Autodesk Inventor part; units mm, degrees
ref_plane "YZ Plane" through (0, 0, 0) normal (1, 0, 0) x (0, 1, 0)
ref_plane "XZ Plane" through (0, 0, 0) normal (0, 1, 0) x (-1, 0, 0)
ref_plane "XY Plane" through (0, 0, 0) normal (0, 0, 1) x (1, 0, 0)
sketch "Sketch1" plane through (0, 0, 0) normal (0, 0, 1) x (1, 0, 0)
  circle A0 centre (0, 0) radius 30
  dimension "d0" = 60
extrude "Extrusion1" add sketch "Sketch1" along normal blind 5
sketch "Sketch2" plane through (0, 0, 5) normal (0, 0, 1) x (1, 0, 0)
  circle A0 centre (0, 0) radius 24.95
  dimension "d3" = 49.9
extrude "Extrusion2" add sketch "Sketch2" along normal blind 5
sketch "Sketch3" plane through (0, 0, 10) normal (0, 0, 1) x (1, 0, 0)
  circle A0 centre (0, 0) radius 15
  dimension "d6" = 30
extrude "Extrusion3" cut sketch "Sketch3" against normal through all
sketch "Sketch4" plane through (0, 0, 0) normal (0, 0, -1) x (-1, 0, 0)
  circle A0 centre (0, 0) radius 20
  dimension "d9" = 40
extrude "Extrusion4" add sketch "Sketch4" against normal blind 5
sketch "Sketch5" plane through (0, 0, 0) normal (0, 0, -1) x (-1, 0, 0)
  circle A0 centre (0, 0) radius 3.5
  dimension "d12" = 7
extrude "Extrusion5" cut sketch "Sketch5" against normal through all
sketch "Sketch6" plane through (0, 0, 5) normal (0, 0, 1) x (1, 0, 0)
  circle A0 centre (7, 0) radius 1.05
  point P0 (0, 0)
  dimension "d15" = 2.1
  dimension "d16" = 7
extrude "Extrusion6" cut sketch "Sketch6" against normal through all
pattern_circular "Circular Pattern1" count 8 over 360 about axis through (0, 0, -10) along (0, 0, 1) of "Extrusion6"
sketch "Sketch9" plane through (0, 0, 0) normal (0, 0, -1) x (-1, 0, 0)
  circle A0 centre (0, 0) radius 15
  circle A1 centre (-4.9497, -4.9497) radius 1.05
  circle A2 centre (0, -7) radius 1.05
  circle A3 centre (4.9497, -4.9497) radius 1.05
  circle A4 centre (7, 0) radius 1.05
  circle A5 centre (4.9497, 4.9497) radius 1.05
  circle A6 centre (0, 7) radius 1.05
  circle A7 centre (-4.9497, 4.9497) radius 1.05
  circle A8 centre (-7, 0) radius 1.05
  circle A9 centre (0, 0) radius 3.5
  circle A10 centre (0, 0) radius 30
  dimension "d35" = 30
extrude "Extrusion9" cut sketch "Sketch9" against normal through all contours A10
sketch "Sketch10" plane through (0, 0, 5) normal (0, 0, 1) x (1, 0, 0)
  circle A0 centre (0, 0) radius 10
  circle A1 centre (4.9497, -4.9497) radius 1.05
  circle A2 centre (0, -7) radius 1.05
  circle A3 centre (-4.9497, -4.9497) radius 1.05
  circle A4 centre (-7, 0) radius 1.05
  circle A5 centre (-4.9497, 4.9497) radius 1.05
  circle A6 centre (0, 7) radius 1.05
  circle A7 centre (4.9497, 4.9497) radius 1.05
  circle A8 centre (7, 0) radius 1.05
  circle A9 centre (0, 0) radius 3.5
  circle A10 centre (0, 0) radius 15
  dimension "d38" = 20
extrude "Extrusion10" add sketch "Sketch10" along normal blind 5 contours A10
sketch "Sketch11" plane through (0, 0, 0) normal (0, 0, -1) x (-1, 0, 0)
  line L0 (-7.5, 0) -> (7.5, 0)
  line L1 (7.5, 0) -> (7.5, -80)
  line L2 (7.5, -80) -> (-7.5, -80)
  line L3 (-7.5, -80) -> (-7.5, 0)
  line L4 (-7.5, 0) -> (7.5, -80) construction
  line L5 (7.5, 0) -> (-7.5, -80) construction
  circle A0 centre (0, 0) radius 15
  circle A1 centre (-4.9497, -4.9497) radius 1.05
  circle A2 centre (0, -7) radius 1.05
  circle A3 centre (4.9497, -4.9497) radius 1.05
  circle A4 centre (7, 0) radius 1.05
  circle A5 centre (4.9497, 4.9497) radius 1.05
  circle A6 centre (0, 7) radius 1.05
  circle A7 centre (-4.9497, 4.9497) radius 1.05
  circle A8 centre (-7, 0) radius 1.05
  circle A9 centre (0, 0) radius 3.5
  line L6 (-15, -75) -> (15, -75)
  line L7 (15, -75) -> (15, -85)
  line L8 (15, -85) -> (-15, -85)
  line L9 (-15, -85) -> (-15, -75)
  line L10 (-15, -75) -> (15, -85) construction
  line L11 (15, -75) -> (-15, -85) construction
  point P0 (0, -40)
  point P1 (7.5, -12.9904)
  point P2 (-7.5, -12.9904)
  point P3 (0, -80)
  point P4 (-7.5, -75)
  point P5 (7.5, -75)
  point P6 (0, 0)
  dimension "d41" = 80
  dimension "d42" = 15
  dimension "d43" = 40
  dimension "d46" = 30
  dimension "d47" = 10
extrude "Extrusion11" add sketch "Sketch11" against normal blind 10 contours A0 L1 L6 L3 | L6 L1 L2 L3 | L3 L2 L1 L6 L7 L8 L9
fillet "Fillet1" radius 5 8 edges at (-7.5, -12.9904, 5) (7.5, -12.9904, 5) (7.5, -75, 5) (15, -75, 5) (15, -85, 5) (-7.5, -75, 5) (-15, -75, 5) (-15, -85, 5)
sketch "Sketch12" plane through (0, 0, 5) normal (0, 0, 1) x (1, 0, 0)
  circle A0 centre (0, 0) radius 4
  dimension "d49" = 8
extrude "Extrusion12" cut sketch "Sketch12" against normal blind 10
properties part number "bearing_bracket3"
Geometry: final body of the model. Coordinates: model frame, mm. A direction names the side the tool comes from. Coordinates: 2 decimals unless noted, no trailing zeros. Write each loop counter-clockwise with the first axis right and the second up, starting at its lowest first coordinate (ties: lowest second). Pieces come first, ordered by that corner, then holes. Notation, with made-up numbers: (-25.5, 64) - (-8.5, 64) arc R19 ccw to (-8.5, 76) - close; hole circle Ø11 at (-28.5, 8.5). An arc over 180 degrees is marked (long way). Return JSON: item names as keys, results as strings.
Item 1: Pin query (flat end, axial travel): pin 1 Ø1.5 at (x, z) = (2.5, 2.5) entering from +Y; pin 2 Ø2.5 at (x, y) = (0, -7) entering from +Z; pin 3 Ø1 at (x, z) = (6, 1) entering from +Y. Return the tip coordinate at first contact, or that it passes through.
Completed:
{"pin 1": "stops at y = 14.9", "pin 2": "stops at z = 5", "pin 3": "stops at y = 13.96"}
Item 2: Section query C-C (y = -47.5). Output: boundary loops of the cut face in (x, z), and give its area (3 significant figures).
Completed:
{"outline": "(-7.5, 0) - (7.5, 0) - (7.5, 10) - (-7.5, 10) - close", "area": "150 mm2"}
Item 3: Line query: L1, parallel to X at y = -33.5, z = 3.5; L2, parallel to X at y = -5.5, z = 7.75; L3, parallel to Y at x = 7, z = 1.3. Output: solid intervals per line, ascending.
Completed:
{"L1": "x = -7.5 to 7.5", "L2": "x = -13.96 to -8.35, 8.35 to 13.96", "L3": "y = -85 to -1.05, 1.05 to 13.27"}
Item 4: Reachability of faces 1 (the face through (-7.5, -42, 5)), 2 (the face through (7.5, -43, 5)), 3 (the face through (-4.3, 0.1, 5)), 4 (the face through (4.12, 5.59, 2.54)) from +Z, -Z, +X, -X, +Y, -Y: full face, straight path, thin tool, end or side. Return the list, or none.
Completed:
{"face 1": "+Z, -Z, -X", "face 2": "+Z, -Z, +X", "face 3": "+Z", "face 4": "+Z, -Z"}
Item 5: Section query A-A (x = 0). Output: boundary loops of the cut face in (y, z).
Completed:
{"outline": "(-85, 0) - (-8.05, 0) - (-8.05, 5) - (-10, 5) - (-10, 10) - (-85, 10) - close; (-5.95, 0) - (-4, 0) - (-4, 5) - (-5.95, 5) - close; (4, 0) - (5.95, 0) - (5.95, 5) - (4, 5) - close; (8.05, 0) - (15, 0) - (15, 10) - (10, 10) - (10, 5) - (8.05, 5) - close"}
Item 6: Section query B-B (y = 0). Output: boundary loops of the cut face in (x, z), and give its area (3 significant figures).
Completed:
{"outline": "(-15, 0) - (-8.05, 0) - (-8.05, 5) - (-10, 5) - (-10, 10) - (-15, 10) - close; (-5.95, 0) - (-4, 0) - (-4, 5) - (-5.95, 5) - close; (4, 0) - (5.95, 0) - (5.95, 5) - (4, 5) - close; (8.05, 0) - (15, 0) - (15, 10) - (10, 10) - (10, 5) - (8.05, 5) - close", "area": "139 mm2"}
Item 7: Section query D-D (z = 3.5). Count the separate pieces of the cut face and the enclosed holes in it, and give its area (3 significant figures).
Completed:
{"separate pieces": "1", "enclosed holes": "9", "area": "1,830 mm2"}
